Verification items for the finished model (mm, model axes). A direction names the side the tool comes from. Round coordinates to 2 decimals unless told otherwise and drop trailing zeros. Order: outer loops, then holes, each group sorted by start corner. A loop starts at its lowest first (then second) coordinate and runs counter-clockwise, first axis right, second up. Notation, with made-up numbers: (57.5, 74) -> (82.5, 74) arc R20 ccw to (82.5, 80) -> close; hole circle Ø10 at (-10, 42.5). An arc over 180 degrees is marked (long way). Put each result on its own line as item: value.
```python
from build123d import *

# Parameters (mm, degrees)
F1_DEPTH = 300
F2_R     = 10
F3_DEPTH = 900.001


with BuildPart() as f1:
    # F0 (on Front) → F1 (new body)
    with BuildSketch(Plane.XZ):
        Polygon((-470.378462, -452.94658), (429.621538, -452.94658), (429.621538, 447.05342), (129.621538, 447.05342), (129.621538, 147.05342), (-170.378462, 147.05342), (-170.378462, -152.94658), (-470.378462, -152.94658), align=None)
    extrude(amount=F1_DEPTH)

    # F2 (on face) → F3 (cut, through all)
    with BuildSketch(Plane.XY.offset(447.05342)):
        with Locations((279.621538, -150)):
            Circle(F2_R)
        with Locations((-10.213119, -150)):
            Circle(F2_R)
        with Locations((-313.667297, -150)):
            Circle(F2_R)
    extrude(amount=-F3_DEPTH, mode=Mode.SUBTRACT)


solid = f1.part
```
Item 1: Material ranges on line 1 along X through (y, z) = (-157.5, -399.5); line 2 along X through (y, z) = (-258, 160); line 3 along Z through (x, y) = (-109, -150.5), recorded low to high.
Geometry check:
line 1: -470.38 to -320.28, -307.05 to -16.83, -3.6 to 273.01, 286.24 to 429.62
line 2: 129.62 to 429.62
line 3: -452.95 to 147.05
Item 2: Sectioned sample at A-A, the plane y = -39. Record the boundary of the cut face in (x, z), then the cut area to 3 significant figures.
Geometry check:
outline: (-470.38, -452.95) -> (429.62, -452.95) -> (429.62, 447.05) -> (129.62, 447.05) -> (129.62, 147.05) -> (-170.38, 147.05) -> (-170.38, -152.95) -> (-470.38, -152.95) -> close
area: 540,000 mm2
Item 3: Sectioned sample at D-D, the plane x = -381.5. Record the boundary of the cut face in (y, z), then the cut area to 3 significant figures.
Geometry check:
outline: (-300, -452.95) -> (0, -452.95) -> (0, -152.95) -> (-300, -152.95) -> close
area: 90,000 mm2
Item 4: Release check for a two-part mould opening along Y. For faces 1 (the face through (-18, -181, 147.053)), 2 (the face through (73, 0, -97)), 3 (the face through (269.63, -149.56, 3.35)) record: pulls with the +Y half, pulls with the -Y half, needs draft (parallel to the pull), parting line crosses it, or undercut.
Geometry check:
face 1: needs draft
face 2: pulls with the +Y half
face 3: undercut
Item 5: Sectioned sample at C-C, the plane z = 243.5. Record the boundary of the cut face in (x, y).
Geometry check:
outline: (129.62, -300) -> (429.62, -300) -> (429.62, 0) -> (129.62, 0) -> close; hole circle Ø20 at (279.62, -150)
Item 6: Sectioned sample at B-B, the plane z = 127. Record the boundary of the cut face in (x, y).
Geometry check:
outline: (-170.38, -300) -> (429.62, -300) -> (429.62, 0) -> (-170.38, 0) -> close; hole circle Ø20 at (-10.21, -150); hole circle Ø20 at (279.62, -150)
Item 7: Tool access check on faces 4 (the face through (-321.603, -156.085, -300.847)), 5 (the face through (-318, -181, -152.947)). Record the directions out of +Z, -Z, +X, -X, +Y, -Y that give a thin tool (end or side, any length) a straight path to the whole face; none if there is none.
Geometry check:
face 4: +Z, -Z
face 5: +Z, -X, +Y, -Y
